Autodesk Inventor part; units mm, degrees
ref_plane "YZ Plane" through (0, 0, 0) normal (1, 0, 0) x (0, 1, 0)
ref_plane "XZ Plane" through (0, 0, 0) normal (0, 1, 0) x (-1, 0, 0)
ref_plane "XY Plane" through (0, 0, 0) normal (0, 0, 1) x (1, 0, 0)
sketch "Sketch_7" plane through (0, 0, 0) normal (0, 0, 1) x (1, 0, 0)
  line L0 (2, 0) -> (-2, 0)
  arc A0 (0, 2.9083) -> (0.0333, 2.875) centre (0.0333, 2.9083) ccw
  line L1 (0.0333, 2.875) -> (0.6693, 2.875)
  arc A1 (1.3307, 2.875) -> (0.6693, 2.875) centre (1, 2.5) ccw
  line L2 (1.3307, 2.875) -> (1.9667, 2.875)
  arc A2 (1.9667, 2.875) -> (2, 2.9083) centre (1.9667, 2.9083) ccw
  line L3 (2, 2.9083) -> (2, 3.4)
  arc A3 (2, 3.4) -> (1.9, 3.5) centre (1.9, 3.4) ccw
  line L4 (1.9, 3.5) -> (0.1, 3.5)
  arc A4 (0.1, 3.5) -> (0, 3.4) centre (0.1, 3.4) ccw
  line L5 (0, 3.4) -> (0, 2.9083)
revolve "Revolution1" add sketch "Sketch_7" angle 360 about axis through (2, 0, 0) along (1, 0, 0)
properties part number "W 618/3_PART2"
Verification items for the finished model (mm, model axes). Round coordinates to 2 decimals unless told otherwise and drop trailing zeros. Order: outer loops, then holes, each group sorted by start corner. A loop starts at its lowest first (then second) coordinate and runs counter-clockwise, first axis right, second up. Notation, with made-up numbers: (31, 34.5) -> (85, 34.5) arc R15 cw to (85, 48.5) -> close; hole circle Ø8 at (60.25, 51.5). An arc over 180 degrees is marked (long way). Put each result on its own line as item: value.
1) Section check A-A (y = 0). Record the cut outline in (x, z) (3 decimals).
Final values:
outline: (0, -3.4) arc R0.1 ccw to (0.1, -3.5) -> (1.9, -3.5) arc R0.1 ccw to (2, -3.4) -> (2, -2.908) arc R0.033 ccw to (1.967, -2.875) -> (1.331, -2.875) arc R0.5 cw to (0.669, -2.875) -> (0.033, -2.875) arc R0.033 ccw to (0, -2.908) -> close; (0, 2.908) arc R0.033 ccw to (0.033, 2.875) -> (0.669, 2.875) arc R0.5 cw to (1.331, 2.875) -> (1.967, 2.875) arc R0.033 ccw to (2, 2.908) -> (2, 3.4) arc R0.1 ccw to (1.9, 3.5) -> (0.1, 3.5) arc R0.1 ccw to (0, 3.4) -> close
2) Section check D-D (x = 1.2). Record the cut outline in (y, z), then the cut area to 3 significant figures.
Final values:
outline: circle Ø7 at (0, 0); hole circle Ø5.92 at (0, 0)
area: 11.0 mm^2
3) Material ranges on line 1 (Z direction, x = 1.7, y = 0) (3 decimals); line 2 (Z direction, x = 1.45, y = -0.5); line 3 (Y direction, x = 0.8, z = -0.25), recorded low to high.
Final values:
line 1: z = -3.5 to -2.875, 2.875 to 3.5
line 2: z = -3.46 to -2.83, 2.83 to 3.46
line 3: y = -3.49 to -2.95, 2.95 to 3.49
4) Section check C-C (x = 1.7). Record the cut outline in (y, z) (3 decimals).
Final values:
outline: circle Ø7 at (0, 0); hole circle Ø5.75 at (0, 0)
5) Mould release check, pull along Y, two halves, no side actions. Record for faces 1 (the cylindrical face through (0.987, 3.233, 1.341)), 2 (the flat face through (0, 3, 1)), 3 (the cylindrical face through (0.36, -0.37, 2.85)): +Y half, -Y half, draft (parallel to the pull), parting line (faces both ways), or undercut.
Final values:
face 1: parting line
face 2: draft
face 3: undercut
6) Depth check by flat-ended pin: pin 1 (1 mm diameter, centred on x = 0.5, y = -1.5, fed in from +Z); pin 2 (2 mm diameter, centred on y = 0.5, z = -0.5, fed in from +X). Enter the tip coordinate at first touch or a pass-through.
Final values:
pin 1: stops at z = 3.35
pin 2: passes through
